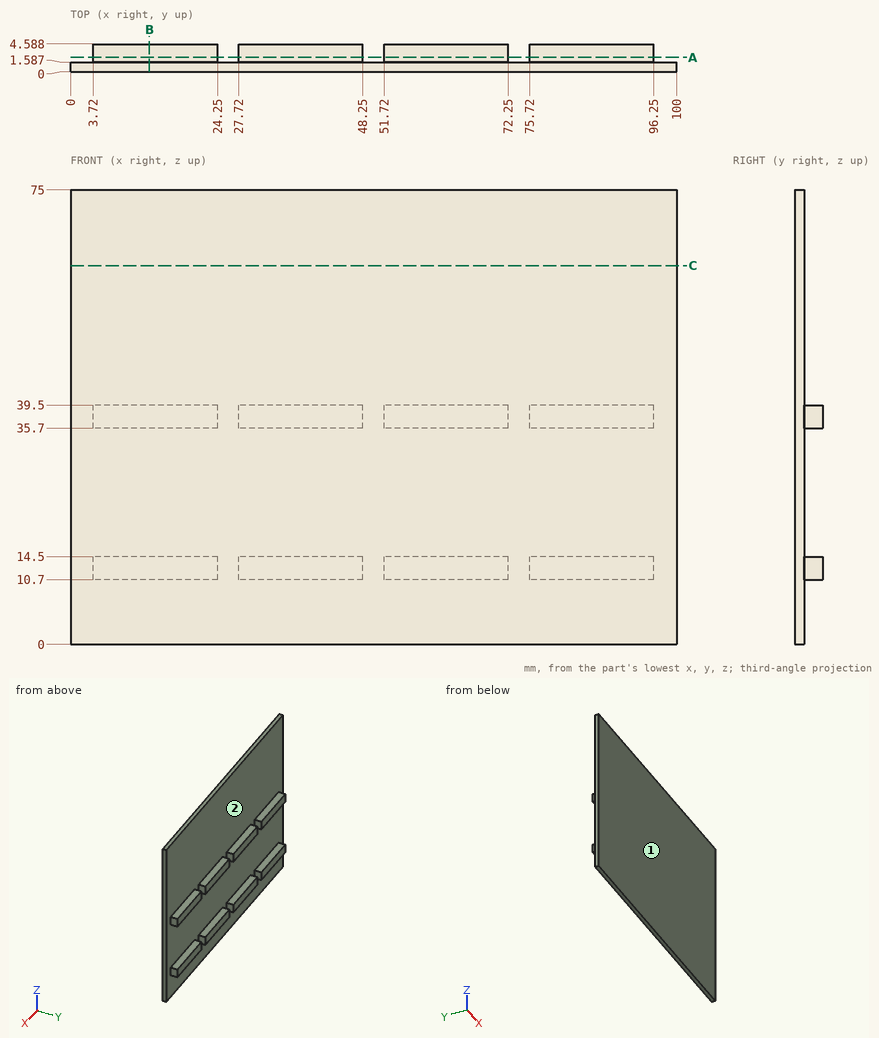
Check sheet for the drawn part. Datum: minimum x, y, z corner. Units: mm. Coordinates: 2 decimals unless noted, no trailing zeros. Write each loop counter-clockwise with the first axis right and the second up, starting at its lowest first coordinate (ties: lowest second). Pieces come first, ordered by that corner, then holes. Notation, with made-up numbers: (8.25, -27) - (53.25, -27) arc R8 ccw to (53.25, -20) - close; hole circle Ø11 at (-37.5, 13.25). An arc over 180 degrees is marked (long way). Answer as a JSON object with one key per item and string values.
(1) Thickness scan on line 1 along X through (y, z) = (2.6, 13); line 2 along Z through (x, y) = (61.5, 3.9); line 3 along Y through (x, z) = (56, 25.5). Record the ranges inside material, lowest first.
Report:
{"line 1": "3.72 to 24.25, 27.72 to 48.25, 51.72 to 72.25, 75.72 to 96.25", "line 2": "10.7 to 14.5, 35.7 to 39.5", "line 3": "0 to 1.59"}
(2) Gauge pin test, flat ends, axial feed: pin 1 Ø1.5 at (y, z) = (3.5, 38) entering from -X; pin 2 Ø0.9 at (x, y) = (66.5, 2.5) entering from -Z; pin 3 Ø1.5 at (x, y) = (15.5, 3) entering from +Z. Record the tip position at first contact, or that the pin passes through.
Report:
{"pin 1": "x = 3.72", "pin 2": "z = 10.7", "pin 3": "z = 39.5"}
(3) Mould release check, pull along Z, two halves, no side actions. Record for the marked faces 1 and 2: pulls with the +Z half, pulls with the -Z half, needs draft (parallel to the pull), parting line crosses it, or undercut.
Report:
{"face 1": "needs draft", "face 2": "undercut"}
(4) Cross-section at C-C on z = 62.5. Record the cut outline in (x, y).
Report:
{"outline": "(0, 0) - (100, 0) - (100, 1.59) - (0, 1.59) - close"}
(5) Cross-section at B-B on x = 13. Record the cut outline in (y, z), plus the area to 3 significant figures.
Report:
{"outline": "(0, 0) - (1.59, 0) - (1.59, 10.7) - (4.59, 10.7) - (4.59, 14.5) - (1.59, 14.5) - (1.59, 35.7) - (4.59, 35.7) - (4.59, 39.5) - (1.59, 39.5) - (1.59, 75) - (0, 75) - close", "area": "142 mm^2"}
(6) Cross-section at A-A on y = 2.4. Give the number of separate pieces and of enclosed holes in the cut face.
Report:
{"separate pieces": "8", "enclosed holes": "0"}
